Check sheet for the modelled part. Datum: model origin and axes. Units: mm. A direction names the side the tool comes from. Round coordinates to 2 decimals unless told otherwise and drop trailing zeros. Loops run counter-clockwise (first coordinate to the right, second up) from the corner with the lowest first, then second, coordinate; pieces in that order, holes last. Notation, with made-up numbers: (-30.75, 45.5) -> (-4.75, 45.5) arc R20 ccw to (-4.75, 61.5) -> close; hole circle Ø9 at (63, 53). An arc over 180 degrees is marked (long way). Use one line per item in the form item = value. Start each with the question number.
(1) Material ranges on probe 1 along X at (y, z) = (1.3, -10); probe 2 along Y at (x, z) = (-32, -2.5); probe 3 along X at (y, z) = (4.2, -7.5), recorded low to high. Write a range as [from, to].
(2) Sectioned sample at C-C (x = -12.5). Record the cut outline in (y, z), and give its area (3 significant figures).
(3) Sectioned sample at D-D (x = -24.5). Record the cut outline in (y, z).
(4) Sectioned sample at B-B (z = -10). Record the cut outline in (x, y), and give its area (3 significant figures).
(5) Sectioned sample at A-A (y = 1.85). Record the cut outline in (x, z), and give its area (3 significant figures).
(6) Draft check along X on faces 1 (the flat face through (-5, 5, -12)), 2 (the flat face through (-48, 5, -18)), 3 (the cylindrical face through (-39.773, 2.028, -10.358)). Enter one of: released by +X, released by -X, zero draft, split by the parting line, or undercut.
(7) Set-up check for faces 4 (the flat face through (-6, 5, -5.036)), 5 (the flat face through (-26, 5, -19.5)), 6 (the flat face through (-7, 5, -11)): record each of +Z, -Z, +X, -X, +Y, -Y from which the full face is reachable in a straight line by a thin tool's end or side.
(8) Go/stop test with flat-tipped pins: pin 1 (0.6 mm diameter, centred on y = 4.5, z = -12, fed in from +X); pin 2 (1.6 mm diameter, centred on x = -25.5, y = 5, fed in from +Z); pin 3 (1 mm diameter, centred on x = -30.5, y = 5, fed in from -Z). Record where each tip stops, or that it passes through.
from build123d import *

# Parameters (mm, degrees)
SKETCH_1_W          = 55
SKETCH_1_H          = 27.5
EXTRUDE_1_DEPTH     = 4
SKETCH_2_R          = 2.75
CUT_EXTRUDE_1_DEPTH = 62.621830547
FILLET_1_R          = 5
SKETCH_4_W          = 20.5
SKETCH_4_H          = 2
SKETCH_4_W_2        = 2
SKETCH_4_H_2        = 12.464207651
EXTRUDE_6_DEPTH     = 2


with BuildPart() as part:
    # 草图1 → 凸台-拉伸1 (new body)
    with BuildSketch(Plane(origin=(0, 0, 0), x_dir=(1, 0, 0), z_dir=(0, 1, 0))):
        with Locations((-27.5, 13.75)):
            Rectangle(SKETCH_1_W, SKETCH_1_H)
    extrude(amount=EXTRUDE_1_DEPTH)

    # 草图2 → 切除-拉伸1 (cut, through all)
    with BuildSketch(Plane(origin=(0, 4, 0), x_dir=(1, 0, 0), z_dir=(0, 1, 0))):
        with Locations(Location((-42.5, 10, 0), (0, 0, 270))):
            Circle(SKETCH_2_R)
        with Locations(Location((-12.5, 10, 0), (0, 0, 270))):
            Circle(SKETCH_2_R)
    extrude(amount=-CUT_EXTRUDE_1_DEPTH, mode=Mode.SUBTRACT)

    # 圆角1
    fillet_1_edges = [part.edges().sort_by_distance(p)[0] for p in [
        (0, 2, 0),
        (-55, 2, 0),
        (-55, 2, -27.5),
        (0, 2, -27.5),
    ]]
    fillet(fillet_1_edges, radius=FILLET_1_R)

    # 草图4 → 凸台-拉伸6 (add)
    with BuildSketch(Plane(origin=(0, 4, 0), x_dir=(1, 0, 0), z_dir=(0, 1, 0))):
        with Locations((-17.25, 18.5)):
            Rectangle(SKETCH_4_W, SKETCH_4_H)
        with Locations((-6, 18.5)):
            Rectangle(SKETCH_4_W_2, SKETCH_4_H)
        with Locations((-6, 11.267896175)):
            Rectangle(SKETCH_4_W_2, SKETCH_4_H_2)
        with Locations((-37.75, 18.5)):
            Rectangle(SKETCH_4_W, SKETCH_4_H)
    extrude(amount=EXTRUDE_6_DEPTH)


solid = part.part
Checks:
q1.probe_1 = [-55, -45.25], [-39.75, -15.25], [-9.75, 0]
q1.probe_2 = [0, 4]
q1.probe_3 = [-7, -5]
q2.outline = (0, -27.5) -> (4, -27.5) -> (4, -19.5) -> (6, -19.5) -> (6, -17.5) -> (4, -17.5) -> (4, -12.75) -> (0, -12.75) -> close; (0, -7.25) -> (4, -7.25) -> (4, 0) -> (0, 0) -> close
q2.area = 92.0 mm2
q3.outline = (0, -27.5) -> (4, -27.5) -> (4, -19.5) -> (6, -19.5) -> (6, -17.5) -> (4, -17.5) -> (4, 0) -> (0, 0) -> close
q4.outline = (-55, 0) -> (-45.25, 0) -> (-45.25, 4) -> (-55, 4) -> close; (-39.75, 0) -> (-15.25, 0) -> (-15.25, 4) -> (-39.75, 4) -> close; (-9.75, 0) -> (0, 0) -> (0, 4) -> (-5, 4) -> (-5, 6) -> (-7, 6) -> (-7, 4) -> (-9.75, 4) -> close
q4.area = 180 mm2
q5.outline = (-55, -22.5) arc R5 ccw to (-50, -27.5) -> (-5, -27.5) arc R5 ccw to (0, -22.5) -> (0, -5) arc R5 ccw to (-5, 0) -> (-50, 0) arc R5 ccw to (-55, -5) -> close; hole circle Ø5.5 at (-42.5, -10); hole circle Ø5.5 at (-12.5, -10)
q5.area = 1,440 mm2
q6.face_1 = released by +X
q6.face_2 = released by -X
q6.face_3 = undercut
q7.face_4 = +Z, +X, -X, +Y
q7.face_5 = -Z, +X, -X, +Y
q7.face_6 = +Z, -X, +Y
q8.pin_1 = -5
q8.pin_2 = -17.5
q8.pin_3 = -19.5
